Answer from the drawing. Dimensions are ordinates in mm from the lowest x, y and z of the part. A direction names the side the tool comes from. Round coordinates to 2 decimals unless told otherwise and drop trailing zeros. Write each loop counter-clockwise with the first axis right and the second up, starting at its lowest first coordinate (ties: lowest second). Pieces come first, ordered by that corner, then holes. Notation, with made-up numbers: (55.25, -40) - (104.25, -40) arc R17 cw to (104.25, -33) - close; hole circle Ø2 at (9, -37). An arc over 180 degrees is marked (long way). One line per item, written item: value. Start each with the question number.
(1) A cutting plane is placed at C-C, the plane z = 23. Determine the outline of the cut face in (x, y), plus the area to 3 significant figures.
(2) A cutting plane is placed at D-D, the plane z = 33. Determine the outline of the cut face in (x, y).
(3) A cutting plane is placed at A-A, the plane x = 27.5. Determine the outline of the cut face in (y, z), plus the area to 3 significant figures.
(4) The mould has two halves that part along Z. Classify the marked faces 4, 5, 6 and 7: +Z half, -Z half, draft (parallel to the pull), parting line (faces both ways), or undercut.
(5) A cutting plane is placed at B-B, the plane y = 4.25. Determine the outline of the cut face in (x, z).
(6) Flat-ended cylindrical pins translate along their axes: pin 1 Ø4 at (x, z) = (27.5, 23) entering from +Y; pin 2 Ø2.5 at (x, z) = (26.5, 60.5) entering from +Y; pin 3 Ø2.5 at (y, z) = (5.5, 57.5) entering from -X; pin 4 Ø4 at (x, y) = (50, 6) entering from -Z. Find the tip coordinate at first contact, or state that the pin passes through.
(7) Find the intervals of material crossed by L1, parallel to Y at x = 42, z = 4.5; L2, parallel to Y at x = 43, z = 27, in increasing order.
(8) For the marked faces 1, 2 and 3, determine the directions among +Z, -Z, +X, -X, +Y, -Y from which every point of the face is accessible in a straight line to the end or side of a thin tool.
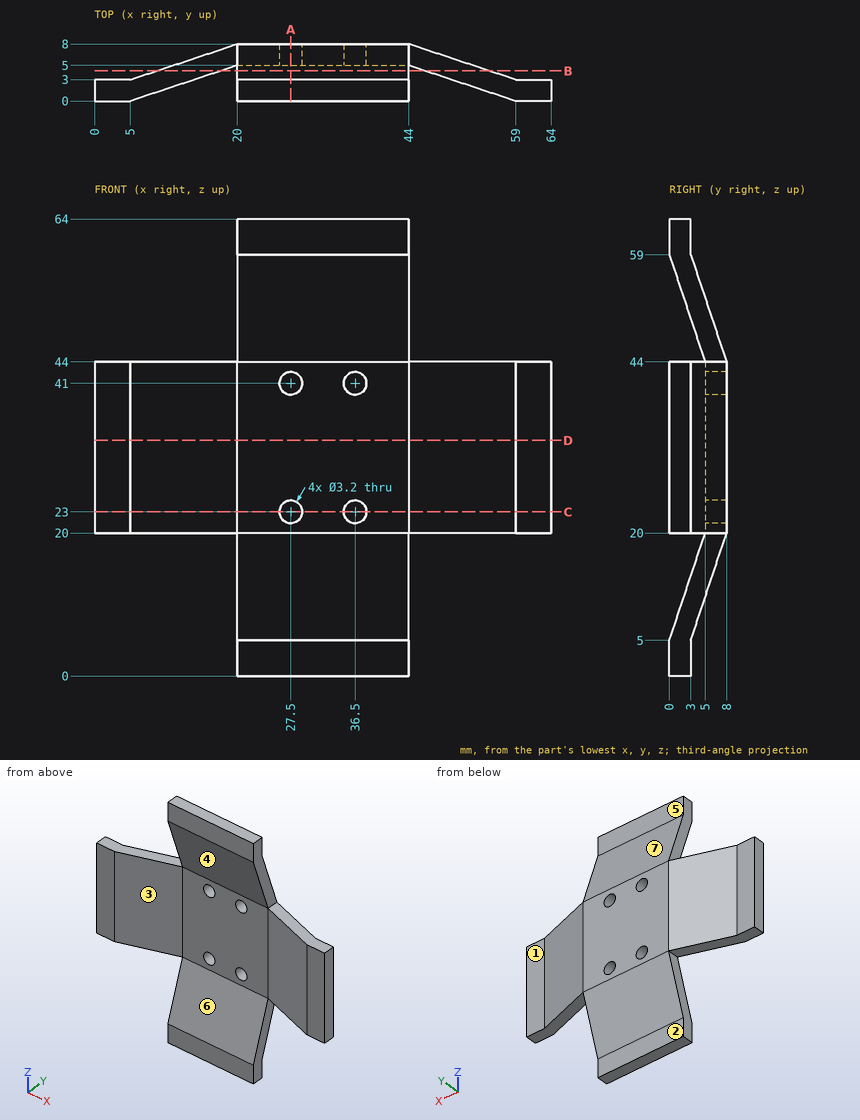
Here are the results:
1. outline: (0, 0) - (5, 0) - (20, 5) - (25.9, 5) - (25.9, 8) - (20, 8) - (5, 3) - (0, 3) - close; (29.1, 5) - (34.9, 5) - (34.9, 8) - (29.1, 8) - close; (38.1, 5) - (44, 5) - (59, 0) - (64, 0) - (64, 3) - (59, 3) - (44, 8) - (38.1, 8) - close
1. area: 173 mm²
2. outline: (0, 0) - (5, 0) - (20, 5) - (44, 5) - (59, 0) - (64, 0) - (64, 3) - (59, 3) - (44, 8) - (20, 8) - (5, 3) - (0, 3) - close
3. outline: (0, 0) - (3, 0) - (3, 5) - (8, 20) - (8, 21.4) - (5, 21.4) - (5, 20) - (0, 5) - close; (0, 59) - (5, 44) - (5, 42.6) - (8, 42.6) - (8, 44) - (3, 59) - (3, 64) - (0, 64) - close; (5, 24.6) - (8, 24.6) - (8, 39.4) - (5, 39.4) - close
3. area: 173 mm²
4. face 4: undercut
4. face 5: draft
4. face 6: undercut
4. face 7: +Z half
5. outline: (8.75, 20) - (17.75, 20) - (17.75, 44) - (8.75, 44) - close; (20, 8.75) - (44, 8.75) - (44, 17.75) - (20, 17.75) - close; (20, 46.25) - (44, 46.25) - (44, 55.25) - (20, 55.25) - close; (46.25, 20) - (55.25, 20) - (55.25, 44) - (46.25, 44) - close
6. pin 1: y = 8
6. pin 2: y = 3
6. pin 3: through
6. pin 4: z = 20
7. L1: 0 to 3
7. L2: 5 to 8
8. face 1: +Z, -Z, +X, +Y
8. face 2: -Z, +X, -X, +Y
8. face 3: +Z, -Z, -Y
